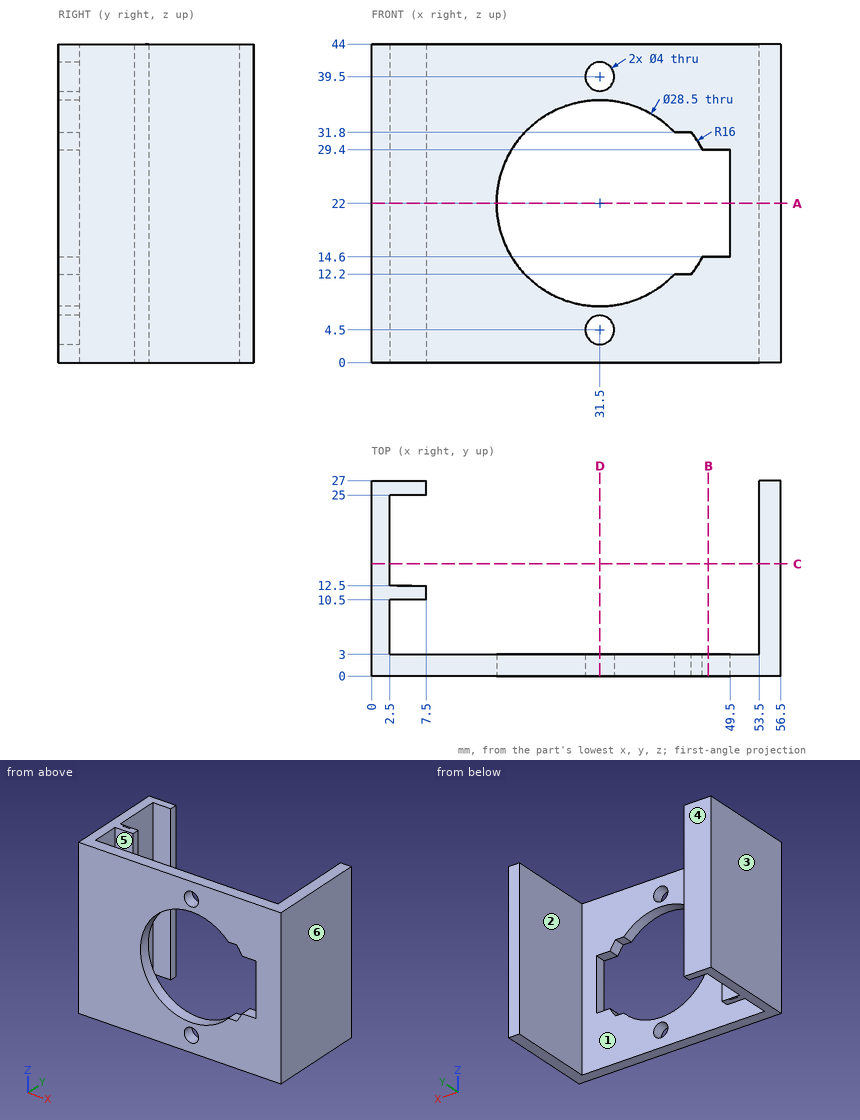
Job drawing, mm, ordinate dimensions from the low corner. One solid piece. A direction names the side the tool comes from. Round coordinates to 2 decimals unless told otherwise and drop trailing zeros. Order: outer loops, then holes, each group sorted by start corner. A loop starts at its lowest first (then second) coordinate and runs counter-clockwise, first axis right, second up. Notation, with made-up numbers: (-3.75, 30.5) -> (25.25, 30.5) arc R34 cw to (25.25, 68.5) -> close; hole circle Ø4 at (7, 8.25). An arc over 180 degrees is marked (long way). Answer in a Markdown table with one row per item.
1) Pin check, flat tips, straight feed: P1, Ø2.5, axis at x = 31.5, z = 39.5, coming from the -Y side; P2, Ø10, axis at x = 46.5, z = 15.5, coming from the +Y side. Stop position of each tip, or through.
Values:
| item | result |
|---|---|
| P1 | through |
| P2 | y = 3 |
2) Band-saw the part on C-C on y = 15.5. Give the cut face in (x, z).
Values:
| item | result |
|---|---|
| outline | (0, 0) -> (2.5, 0) -> (2.5, 44) -> (0, 44) -> close; (53.5, 0) -> (56.5, 0) -> (56.5, 44) -> (53.5, 44) -> close |
3) Mould opens along X. For the marked faces 4, 5 and 6 say: released by +X, released by -X, zero draft, split by the parting line, or undercut.
Values:
| item | result |
|---|---|
| face 4 | zero draft |
| face 5 | undercut |
| face 6 | released by +X |
4) Which spindle directions (+Z, -Z, +X, -X, +Y, -Y) get a long thin tool onto all of the face, cutting with end or side? Do the marked faces 1, 2 and 3. Say none if no direction does.
Values:
| item | result |
|---|---|
| face 1 | +Z, -Z |
| face 2 | +Z, -Z, +Y |
| face 3 | +Z, -Z, -X, +Y, -Y |
5) Band-saw the part on D-D on x = 31.5. Give the cut face in (y, z).
Values:
| item | result |
|---|---|
| outline | (0, 0) -> (3, 0) -> (3, 2.5) -> (0, 2.5) -> close; (0, 6.5) -> (3, 6.5) -> (3, 7.75) -> (0, 7.75) -> close; (0, 36.25) -> (3, 36.25) -> (3, 37.5) -> (0, 37.5) -> close; (0, 41.5) -> (3, 41.5) -> (3, 44) -> (0, 44) -> close |
6) Wall check: L1, parallel to Y at x = 7, z = 33.5; L2, parallel to X at y = 2.25, z = 39.5; L3, parallel to X at y = 24.75, z = 10. Give the ranges that are in metal, low to high.
Values:
| item | result |
|---|---|
| L1 | 0 to 3, 10.5 to 12.5, 25 to 27 |
| L2 | 0 to 29.5, 33.5 to 56.5 |
| L3 | 0 to 2.5, 53.5 to 56.5 |
7) Band-saw the part on A-A on z = 22. Give the cut face in (x, y).
Values:
| item | result |
|---|---|
| outline | (0, 0) -> (17.25, 0) -> (17.25, 3) -> (2.5, 3) -> (2.5, 10.5) -> (7.5, 10.5) -> (7.5, 12.5) -> (2.5, 12.5) -> (2.5, 25) -> (7.5, 25) -> (7.5, 27) -> (0, 27) -> close; (49.5, 0) -> (56.5, 0) -> (56.5, 27) -> (53.5, 27) -> (53.5, 3) -> (49.5, 3) -> close |
8) Band-saw the part on B-B on x = 46.5. Give the cut face in (y, z).
Values:
| item | result |
|---|---|
| outline | (0, 0) -> (3, 0) -> (3, 14.6) -> (0, 14.6) -> close; (0, 29.4) -> (3, 29.4) -> (3, 44) -> (0, 44) -> close |
